The model under review builds one solid part; all positions refer to its coordinate system, in mm. Face numbers are marked on the shaded views. A direction names the side the tool comes from. Round coordinates to 2 decimals unless told otherwise and drop trailing zeros. Loops run counter-clockwise (first coordinate to the right, second up) from the corner with the lowest first, then second, coordinate; pieces in that order, holes last. Notation, with made-up numbers: (69.25, -24.5) -> (96.25, -24.5) arc R9 cw to (96.25, -19.5) -> close; hole circle Ø8 at (85.25, 25.25). An arc over 180 degrees is marked (long way). Return JSON: item names as keys, results as strings. Group by question number.
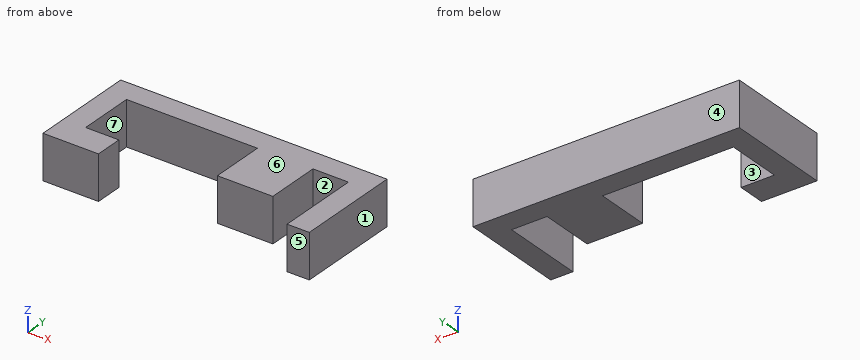
```python
from build123d import *

# Parameters (mm, degrees)
BOX003_W     = 85
BOX003_H     = 13
BOX003_DEPTH = 20
BOX002_W     = 16
BOX002_H     = 25
BOX002_DEPTH = 20
BOX001_W     = 59
BOX001_H     = 25
BOX001_DEPTH = 20
BOX_W        = 120
BOX_H        = 47.5
BOX_DEPTH    = 20


with BuildPart() as cube003:
    # Box003 → Box003 (new body)
    with BuildSketch(Plane(origin=(25, 0, 0), x_dir=(1, 0, 0), z_dir=(0, 0, 1))):
        with Locations((42.5, 6.5)):
            Rectangle(BOX003_W, BOX003_H)
    extrude(amount=BOX003_DEPTH)


with BuildPart() as cube002:
    # Box002 → Box002 (new body)
    with BuildSketch(Plane(origin=(94, 12.5, 0), x_dir=(1, 0, 0), z_dir=(0, 0, 1))):
        with Locations((8, 12.5)):
            Rectangle(BOX002_W, BOX002_H)
    extrude(amount=BOX002_DEPTH)


with BuildPart() as cube001:
    # Box001 → Box001 (new body)
    with BuildSketch(Plane(origin=(10, 12.5, 0), x_dir=(1, 0, 0), z_dir=(0, 0, 1))):
        with Locations((29.5, 12.5)):
            Rectangle(BOX001_W, BOX001_H)
    extrude(amount=BOX001_DEPTH)


with BuildPart() as cut002:
    # Box → Box (new body)
    with BuildSketch(Plane.XY):
        with Locations((60, 23.75)):
            Rectangle(BOX_W, BOX_H)
    extrude(amount=BOX_DEPTH)

    # Cut: cut Cube001
    add(cube001.part, mode=Mode.SUBTRACT)

    # Cut001: cut Cube002
    add(cube002.part, mode=Mode.SUBTRACT)

    # Cut002: cut Cube003
    add(cube003.part, mode=Mode.SUBTRACT)


solid = cut002.part
```
1. We need section D-D, the plane x = 104. Write out the cut boundary in (y, z), then the cut area to 3 significant figures.
2. Wall thickness on line 1 (X direction, y = 30.5, z = 2.5); line 2 (Y direction, x = 22, z = 10); line 3 (X direction, y = 8.5, z = 6.75): over which ranges is each line inside the solid? List them lowest first.
3. We need section A-A, the plane y = 33.5. Write out the cut boundary in (x, z), then the cut area to 3 significant figures.
4. Tool access review of the marked faces 1, 2 and 3: name each direction out of +Z, -Z, +X, -X, +Y, -Y from which nothing blocks a thin tool from reaching the whole face with its end or side.
5. For P1, Ø5, axis at x = 62, z = 12.5, coming from the -Y side; P2, Ø6, axis at x = 78.5, z = 7, coming from the -Y side, all flat-tipped, find the tip position at first contact; note any pin that passes through.
6. We need section C-C, the plane z = 3.75. Write out the cut boundary in (x, y).
7. We need section B-B, the plane y = 10. Write out the cut boundary in (x, z), then the cut area to 3 significant figures.
8. Draft analysis for pull direction Y (two halves, no side actions). For the marked faces 4, 5, 6 and 7, state which applies: pulls with the +Y half, pulls with the -Y half, needs draft (parallel to the pull), parting line crosses it, or undercut.
Check sheet entries:
{
 "1": {"outline": "(37.5, 0) -> (47.5, 0) -> (47.5, 20) -> (37.5, 20) -> close", "area": "200 mm²"},
 "2": {"line 1": "x = 0 to 10, 69 to 94, 110 to 120", "line 2": "y = 0 to 12.5, 37.5 to 47.5", "line 3": "x = 0 to 25, 110 to 120"},
 "3": {"outline": "(0, 0) -> (10, 0) -> (10, 20) -> (0, 20) -> close; (69, 0) -> (94, 0) -> (94, 20) -> (69, 20) -> close; (110, 0) -> (120, 0) -> (120, 20) -> (110, 20) -> close", "area": "900 mm²"},
 "4": {"face 1": "+Z, -Z, +X, +Y, -Y", "face 2": "+Z, -Z, -Y", "face 3": "+Z, -Z"},
 "5": {"P1": "stops at y = 37.5", "P2": "stops at y = 13"},
 "6": {"outline": "(0, 0) -> (25, 0) -> (25, 12.5) -> (10, 12.5) -> (10, 37.5) -> (69, 37.5) -> (69, 13) -> (94, 13) -> (94, 37.5) -> (110, 37.5) -> (110, 0) -> (120, 0) -> (120, 47.5) -> (0, 47.5) -> close"},
 "7": {"outline": "(0, 0) -> (25, 0) -> (25, 20) -> (0, 20) -> close; (110, 0) -> (120, 0) -> (120, 20) -> (110, 20) -> close", "area": "700 mm²"},
 "8": {"face 4": "pulls with the +Y half", "face 5": "pulls with the -Y half", "face 6": "needs draft", "face 7": "undercut"}
}
